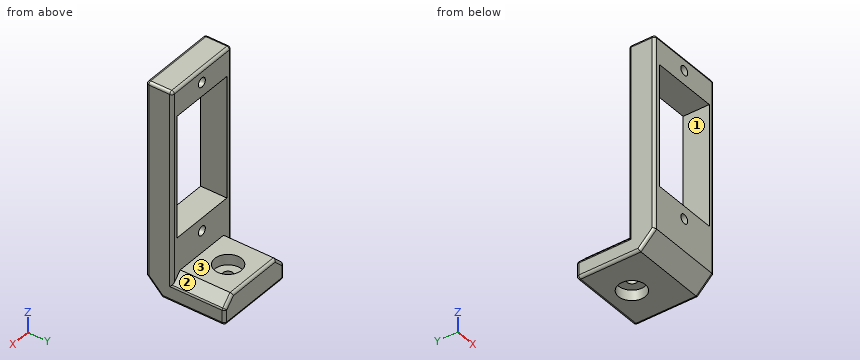
Autodesk Fusion 360 part; units mm, degrees
sketch "Sketch1" plane through (0, 0, 0) normal (0, 0, 1) x (1, 0, 0)
  line L0 (0, 0) -> (15, 0)
  line L1 (15, 0) -> (15, 15)
  line L2 (15, 15) -> (0, 15)
  line L3 (0, 15) -> (0, 0)
  line L4 (0, 0) -> (15, 0)
  line L5 (15, 0) -> (15, 5)
  line L6 (15, 5) -> (0, 5)
  line L7 (0, 5) -> (0, 0)
  dimension "d1" = 15
  dimension "d2" = 15
extrude "Extrude1" add sketch "Sketch1" along normal blind 5 contours L1 L2 L3 L6
extrude "Extrude2" add sketch "Sketch1" along normal blind 40 contours L0 L1 L3 L4 L5 L6 L7
sketch "Sketch2" plane through (0, 5, 0) normal (0, 1, 0) x (-1, 0, 0)
  line L0 (-15, 5) -> (0, 5)
  line L1 (0, 5) -> (0, 40)
  line L2 (0, 40) -> (-15, 40)
  line L3 (-15, 40) -> (-15, 5)
  line L4 (-13.85, 11.6) -> (-13.85, 34.85)
  line L5 (-1.15, 11.6) -> (-13.85, 11.6)
  circle A0 centre (-7.5, 9.15) radius 0.875
  line L6 (-1.15, 34.85) -> (-1.15, 11.6)
  circle A1 centre (-7.5, 37.5) radius 0.875
  line L7 (-13.85, 34.85) -> (-1.15, 34.85)
  dimension "d7" = 23.25
  dimension "d8" = 12.7
  dimension "d9" = 1.75
  dimension "d10" = 1.75
  dimension "d11" = 2.45
  dimension "d12" = 2.65
  dimension "d13" = 1.15
  dimension "d14" = 2.5
extrude "Extrude3" cut sketch "Sketch2" against normal blind 5 contours L4 L5 L6 L7 | A0 | A1
sketch "Sketch3" plane through (0, 0, 5) normal (0, 0, 1) x (-1, 0, 0)
  line L0 (-15, -15) -> (0, -15)
  line L1 (0, -15) -> (0, -5)
  line L2 (0, -5) -> (-15, -5)
  line L3 (-15, -5) -> (-15, -15)
  circle A0 centre (-7.5, -10) radius 0.95
  circle A1 centre (-7.5, -10) radius 2.55
  line L4 (-15, -15) -> (0, -15)
  dimension "d17" = 5.1
  dimension "d18" = 1.9
  dimension "d19" = 7.5
  dimension "d20" = 5
extrude "Extrude4" cut sketch "Sketch3" against normal blind 5 contours A0 | A1
extrude "Extrude7" add sketch "Sketch3" against normal blind 3 contours A1
extrude "Extrude8" cut sketch "Sketch3" against normal blind 2 contours A1
chamfer "Chamfer2" distance 3 angle 45 1 edges at (7.5, 0, 0)
chamfer "Chamfer3" distance 2 angle 45 2 edges at (15, 10, 5) (0, 10, 5)
fillet "Fillet4" radius 0.5 4 faces at (5, 3.3333, 40) (15, 1.6667, 16) (0, 3.3333, 27.6667) (9.3333, 15, 1.6667)
fillet "Fillet3" [suppressed]
Model file for the job. Use its own axes, mm. Face numbers are marked on the shaded views. A direction names the side the tool comes from. Coordinates: 2 decimals unless noted, no trailing zeros. Loops run counter-clockwise (first coordinate to the right, second up) from the corner with the lowest first, then second, coordinate; pieces in that order, holes last. Notation, with made-up numbers: (35.25, -15.5) - (67.25, -15.5) arc R20 ccw to (67.25, 21.5) - close; hole circle Ø10 at (27.5, 14.25). An arc over 180 degrees is marked (long way). Answer as a JSON object with one key per item and string values. Group by question number.
(1) Cut at A-A (z = 26). Give the cut face in (x, y).
(2) Cut at D-D (z = 37.5). Give the cut face in (x, y) (3 decimals).
(3) Cut at C-C (x = 11). Give the cut face in (y, z).
(4) Cut at B-B (y = 10). Give the cut face in (x, z).
(5) Flat gauge pins, fed straight in: pin 1 (8 mm diameter, centred on x = 7.5, y = 10, fed in from +Z); pin 2 (2.5 mm diameter, centred on x = 7.5, y = 10, fed in from +Z); pin 3 (4 mm diameter, centred on x = 7.5, y = 10, fed in from -Z); pin 4 (1.6 mm diameter, centred on x = 7.5, z = 37.5, fed in from -Y). Where does each tip first touch, or does it go through?
(6) Probe line 1 along X through (y, z) = (2.75, 26.5); line 2 along Y through (x, z) = (7.5, 3.95); line 3 along Y through (x, z) = (7.5, 2.5). List the from-to ranges inside material, lowest first.
(7) Tool access for the marked faces 1, 2 and 3: list every direction of +Z, -Z, +X, -X, +Y, -Y with a clear straight run to the whole face (end or side of a thin tool).
Geometry says:
{
 "1": {"outline": "(0, 0.5) arc R0.5 ccw to (0.5, 0) - (1.15, 0) - (1.15, 5) - (0.5, 5) arc R0.5 ccw to (0, 4.5) - close; (13.85, 0) - (14.5, 0) arc R0.5 ccw to (15, 0.5) - (15, 4.5) arc R0.5 ccw to (14.5, 5) - (13.85, 5) - close"},
 "2": {"outline": "(0, 0.5) arc R0.5 ccw to (0.5, 0) - (6.625, 0) - (6.625, 5) - (0.5, 5) arc R0.5 ccw to (0, 4.5) - close; (8.375, 0) - (14.5, 0) arc R0.5 ccw to (15, 0.5) - (15, 4.5) arc R0.5 ccw to (14.5, 5) - (8.375, 5) - close"},
 "3": {"outline": "(0, 3) - (3, 0) - (14.5, 0) arc R0.5 ccw to (15, 0.5) - (15, 4.5) arc R0.5 ccw to (14.5, 5) - (5, 5) - (5, 11.6) - (0, 11.6) - close; (0, 34.85) - (5, 34.85) - (5, 39.5) arc R0.5 ccw to (4.5, 40) - (0.5, 40) arc R0.5 ccw to (0, 39.5) - close"},
 "4": {"outline": "(0, 0.5) arc R0.5 ccw to (0.5, 0) - (4.95, 0) - (4.95, 2) - (6.55, 2) - (6.55, 3) - (4.95, 3) - (4.95, 5) - (2, 5) - (0.15, 3.15) arc R0.5 ccw to (0, 2.79) - close; (8.45, 2) - (10.05, 2) - (10.05, 0) - (14.5, 0) arc R0.5 ccw to (15, 0.5) - (15, 2.79) arc R0.5 ccw to (14.85, 3.15) - (13, 5) - (10.05, 5) - (10.05, 3) - (8.45, 3) - close"},
 "5": {"pin 1": "stops at z = 5", "pin 2": "stops at z = 3", "pin 3": "stops at z = 2", "pin 4": "passes through"},
 "6": {"line 1": "x = 0 to 1.15, 13.85 to 15", "line 2": "y = 0 to 7.45, 12.55 to 15", "line 3": "y = 0.5 to 9.05, 10.95 to 15"},
 "7": {"face 1": "+Y, -Y", "face 2": "+Z, +X, +Y", "face 3": "+Z, +X, -X, +Y"}
}
